Read the model definition and answer for the solid it produces. Units are mm, in the model's axes. Round coordinates to 2 decimals unless told otherwise and drop trailing zeros. Write each loop counter-clockwise with the first axis right and the second up, starting at its lowest first coordinate (ties: lowest second). Pieces come first, ordered by that corner, then holes. Notation, with made-up numbers: (66.25, 34) - (108.25, 34) arc R30 cw to (108.25, 59) - close; hole circle Ø3 at (58, -13.5). An arc over 180 degrees is marked (long way). One line per item, written item: value. Start each with the question number.
(1) A cutting plane is placed at C-C, the plane x = 12.5. State how many separate pieces and enclosed holes the cut face has, plus the area to 3 significant figures.
(2) Find the intervals of material crossed by L1, parallel to Y at x = 13.5, z = 38.5; L2, parallel to Z at x = 10.5, y = 177.8; L3, parallel to Y at x = 8, z = 46, in increasing order.
(3) A cutting plane is placed at B-B, the plane z = 25. Determine the outline of the cut face in (x, y) (1 decimal), plus the area to 3 significant figures.
(4) A flat-ended cylindrical pin translates along its axis: pin 1 Ø1.7 at (y, z) = (80.5, 45.5) entering from +X. Find the tip coordinate at first contact, or state that the pin passes through.
(5) A cutting plane is placed at A-A, the plane y = 152.4. Determine the outline of the cut face in (x, z) (1 decimal), plus the area to 3 significant figures.
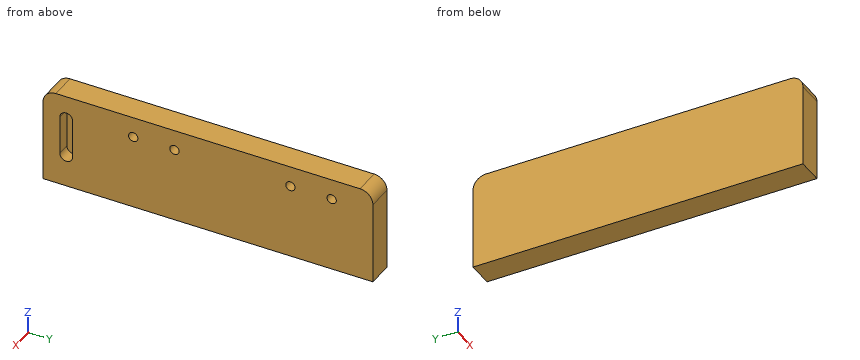
from build123d import *

# Parameters (mm, degrees)
F1_DEPTH = 15.875
F2_R     = 2.875
F3_DEPTH = 7.9375


with BuildPart() as f1:
    # F0 (on Right) → F1 (new body)
    with BuildSketch(Plane.YZ):
        with BuildLine():
            Line((0, 50.8), (0, 0))
            Line((0, 0), (203.2, 0))
            Line((203.2, 0), (203.2, 50.8))
            ThreePointArc((203.2, 50.8), (200.87516, 56.41266), (195.2625, 58.7375))
            Line((195.2625, 58.7375), (7.9375, 58.7375))
            ThreePointArc((7.9375, 58.7375), (2.32484, 56.41266), (0, 50.8))
        make_face()
    extrude(amount=F1_DEPTH)

    # F2 (on face) → F3 (cut)
    with BuildSketch(Plane.YZ.offset(15.875)):
        with BuildLine():
            ThreePointArc((18.25625, 44.053125), (14.2875, 48.021875), (10.31875, 44.053125))
            Line((10.31875, 44.053125), (10.31875, 20.240625))
            ThreePointArc((10.31875, 20.240625), (14.2875, 16.271875), (18.25625, 20.240625))
            Line((18.25625, 20.240625), (18.25625, 44.053125))
        make_face()
        with Locations((55.5625, 46.0375)):
            Circle(F2_R)
        with Locations((80.9625, 46.0375)):
            Circle(F2_R)
        with Locations((152.4, 46.0375)):
            Circle(F2_R)
        with Locations((177.8, 46.0375)):
            Circle(F2_R)
    extrude(amount=-F3_DEPTH, mode=Mode.SUBTRACT)


solid = f1.part
Here are the results:
1. separate pieces: 1
1. enclosed holes: 5
1. area: 11,600 mm²
2. L1: 0 to 10.32, 18.26 to 203.2
2. L2: 0 to 43.16, 48.91 to 58.74
2. L3: 0 to 10.83, 17.75 to 52.69, 58.44 to 78.09, 83.84 to 149.53, 155.27 to 174.93, 180.67 to 203.2
3. outline: (0, 0) - (15.9, 0) - (15.9, 10.3) - (7.9, 10.3) - (7.9, 18.3) - (15.9, 18.3) - (15.9, 203.2) - (0, 203.2) - close
3. area: 3,160 mm²
4. pin 1: x = 7.94
5. outline: (0, 0) - (15.9, 0) - (15.9, 43.2) - (7.9, 43.2) - (7.9, 48.9) - (15.9, 48.9) - (15.9, 58.7) - (0, 58.7) - close
5. area: 887 mm²
